The model under review builds one solid part; all positions refer to its coordinate system, in mm. Face numbers are marked on the shaded views. A direction names the side the tool comes from. Coordinates: 2 decimals unless noted, no trailing zeros. Order: outer loops, then holes, each group sorted by start corner. A loop starts at its lowest first (then second) coordinate and runs counter-clockwise, first axis right, second up.
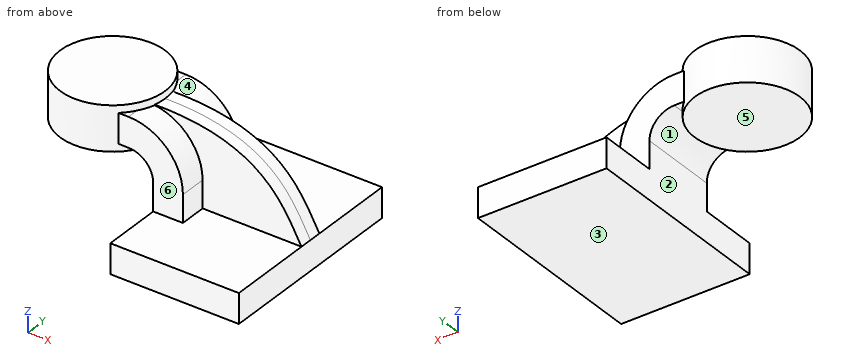
from build123d import *

# Parameters (mm, degrees)
F1_DEPTH = 63.5
F0_W     = 17.08876
F0_H     = 4.7498
F2_DEPTH = 25.4
F3_DEPTH = 7.9375


with BuildPart() as f1:
    # F0 (on Front) → F1 (new body, symmetric)
    with BuildSketch(Plane.XZ):
        Polygon((-41.275, 9.525), (-41.275, -9.525), (41.275, -9.525), (41.275, 9.525), (-22.225, 9.525), align=None)
    extrude(amount=F1_DEPTH, both=True)

    # F0 (on Front) → F2 (join, symmetric)
    with BuildSketch(Plane.XZ):
        with Locations((-77.18062, 64.3001)):
            Rectangle(F0_W, F0_H)
        with BuildLine():
            Line((-41.275, 27.0002), (-41.275, 9.525))
            Line((-41.275, 9.525), (-22.225, 9.525))
            Line((-22.225, 9.525), (-22.225, 27.0002))
            ThreePointArc((-22.225, 27.0002), (-32.454296, 51.695904), (-57.15, 61.9252))
            Line((-57.15, 61.9252), (-68.63624, 61.9252))
            Line((-68.63624, 61.9252), (-68.63624, 42.8752))
            Line((-68.63624, 42.8752), (-57.15, 42.8752))
            ThreePointArc((-57.15, 42.8752), (-45.92468, 38.22552), (-41.275, 27.0002))
        make_face()
    extrude(amount=F2_DEPTH, both=True)

    # F0 (on Front) → F3 (join, symmetric)
    with BuildSketch(Plane.XZ):
        with BuildLine():
            Line((-22.225, 9.525), (41.275, 9.525))
            add(Edge.make_bspline(
                [(41.275, 9.525), (30.298301, 28.204535), (17.943603, 64.763766), (-57.15, 61.9252)],
                knots=[0, 0, 0, 0, 111.504536, 111.504536, 111.504536, 111.504536], degree=3))
            ThreePointArc((-57.15, 61.9252), (-32.454296, 51.695904), (-22.225, 27.0002))
            Line((-22.225, 27.0002), (-22.225, 9.525))
        make_face()
    extrude(amount=F3_DEPTH, both=True)

    # F0 (on Front) → F4 (revolve)
    with BuildSketch(Plane.XZ):
        Polygon((-85.725, 42.8752), (-85.725, 61.9252), (-85.725, 66.675), (-119.43624, 66.675), (-119.43624, 38.1), (-85.725, 38.1), align=None)
    revolve(axis=Axis((-85.725, 0, 52.3875), (0, 0, 1)))


solid = f1.part
(1) The part is to be moulded in two halves that separate along X. For the marked faces 1, 2 and 3, say which applies: +X half, -X half, draft (parallel to the pull), parting line (faces both ways), or undercut.
(2) Wall thickness on line 1 (Z direction, x = -103.5, y = -25) (3 decimals); line 2 (X direction, y = 18, z = 18) (3 decimals); line 3 (Z direction, x = 11.5, y = -31) (3 decimals): over which ranges is each line inside the solid? List them lowest first.
(3) Consider section C-C (y = 10). Give the boundary of the cut face in (x, z) (3 decimals), then the cut area to 3 significant figures.
(4) Tool access review of the marked faces 4, 5 and 6: name each direction out of +Z, -Z, +X, -X, +Y, -Y from which nothing blocks a thin tool from reaching the whole face with its end or side.
(5) Consider section B-B (y = 55). Give the boundary of the cut face in (x, z) (3 decimals).
(6) Consider section A-A (y = -29.5). Give the boundary of the cut face in (x, z) (3 decimals), then the cut area to 3 significant figures.
(7) Insertion check: pin 1 Ø1.9 at (x, y) = (-61.5, -20) entering from -Z; pin 2 Ø3 at (x, y) = (-60.5, -23.5) entering from +Z (3 decimals); pin 3 Ø4 at (x, z) = (-80.5, 42.5) entering from +Y; pin 4 Ø14 at (y, z) = (-17.5, 18) entering from +X (3 decimals). Each pin has a flat end and moves straight along its axis. Give the tip position at first contact, or say it passes through.
Findings:
1. face 1: undercut
1. face 2: -X half
1. face 3: draft
2. line 1: z = 38.1 to 66.675
2. line 2: x = -41.275 to -22.225
2. line 3: z = -9.525 to 9.525
3. outline: (-117.919, 38.1) - (-53.531, 38.1) - (-53.531, 42.457) arc R15.875 cw to (-41.275, 27) - (-41.275, -9.525) - (41.275, -9.525) - (41.275, 9.525) - (-22.225, 9.525) - (-22.225, 27) arc R34.925 ccw to (-53.531, 61.737) - (-53.531, 66.675) - (-117.919, 66.675) - close
3. area: 4,440 mm2
4. face 4: +Z, +X, +Y
4. face 5: -Z, -X, +Y, -Y
4. face 6: +Z, +X, -Y
5. outline: (-41.275, -9.525) - (41.275, -9.525) - (41.275, 9.525) - (-41.275, 9.525) - close
6. outline: (-102.041, 38.1) - (-69.409, 38.1) - (-69.409, 66.675) - (-102.041, 66.675) - close; (-41.275, -9.525) - (41.275, -9.525) - (41.275, 9.525) - (-41.275, 9.525) - close
6. area: 2,510 mm2
7. pin 1: stops at z = 38.1
7. pin 2: stops at z = 66.675
7. pin 3: stops at y = 33.56
7. pin 4: stops at x = -22.225
